```python
from build123d import *

# Parameters (mm, degrees)
SKETCH1_W           = 25.4
SKETCH1_H           = 38.1
BOSS_EXTRUDE1_DEPTH = 152.4
SHELL1_T            = -3.175
SKETCH2_R           = 9.525
CUT_EXTRUDE1_DEPTH  = 156.672163536
SKETCH3_R           = 2.38125
CUT_EXTRUDE2_DEPTH  = 158.602855304
SKETCH4_R           = 2.38125
CUT_EXTRUDE3_DEPTH  = 156.672163536
SKETCH5_R           = 2.38125
CUT_EXTRUDE4_DEPTH  = 158.602855304


with BuildPart() as part:
    # Sketch1 → Boss-Extrude1 (new body)
    with BuildSketch(Plane.XY):
        Rectangle(SKETCH1_W, SKETCH1_H)
    extrude(amount=BOSS_EXTRUDE1_DEPTH)

    # Shell1
    shell1_openings = [part.faces().sort_by_distance(p)[0] for p in [
        (0, 0, 152.4),
        (0, 0, 0),
    ]]
    offset(amount=SHELL1_T, openings=shell1_openings, kind=Kind.INTERSECTION)

    # Sketch2 → Cut-Extrude1 (cut, through all)
    with BuildSketch(Plane(origin=(12.7, 0, 0), x_dir=(0, 0, -1), z_dir=(1, 0, 0))):
        with Locations((-53.975, -12.7)):
            Circle(SKETCH2_R)
    extrude(amount=-CUT_EXTRUDE1_DEPTH, mode=Mode.SUBTRACT)

    # Sketch3 → Cut-Extrude2 (cut, through all)
    with BuildSketch(Plane(origin=(0, 19.05, 0), x_dir=(1, 0, 0), z_dir=(0, 1, 0))):
        with Locations(Location((0, -139.7, 0), (0, 0, 270))):
            Circle(SKETCH3_R)
        with Locations(Location((0, -114.3, 0), (0, 0, 270))):
            Circle(SKETCH3_R)
    extrude(amount=-CUT_EXTRUDE2_DEPTH, mode=Mode.SUBTRACT)

    # Sketch4 → Cut-Extrude3 (cut, through all)
    with BuildSketch(Plane(origin=(12.7, 0, 0), x_dir=(0, 0, -1), z_dir=(1, 0, 0))):
        with Locations(Location((-79.375, -9.525, 0), (0, 0, 90))):
            Circle(SKETCH4_R)
        with Locations(Location((-104.775, -9.525, 0), (0, 0, 90))):
            Circle(SKETCH4_R)
    extrude(amount=-CUT_EXTRUDE3_DEPTH, mode=Mode.SUBTRACT)

    # Sketch5 → Cut-Extrude4 (cut, through all)
    with BuildSketch(Plane(origin=(0, 19.05, 0), x_dir=(1, 0, 0), z_dir=(0, 1, 0))):
        with Locations(Location((0, -12.7, 0), (0, 0, 270))):
            Circle(SKETCH5_R)
        with Locations(Location((0, -38.1, 0), (0, 0, 270))):
            Circle(SKETCH5_R)
    extrude(amount=-CUT_EXTRUDE4_DEPTH, mode=Mode.SUBTRACT)


solid = part.part
```
Read the model definition and answer for the solid it produces. Units are mm, in the model's axes. A direction names the side the tool comes from. Give positions to 0.01 mm unless a question says otherwise; leave off trailing zeros. Loops run counter-clockwise (first coordinate to the right, second up) from the corner with the lowest first, then second, coordinate; pieces in that order, holes last.
Item 1: The part is cut by section C-C (y = 11.5). Write down the section's boundary in (x, z) (3 decimals).
Item 2: The part is cut by section D-D (y = -9.5). Give the number of separate pieces and of enclosed holes in the cut face, and give its area (3 significant figures).
Item 3: Find the intervals of material crossed by line 1 along X through (y, z) = (14, 61) (3 decimals); line 2 along Y through (x, z) = (-9, 67) (3 decimals); line 3 along X through (y, z) = (17, 38), in increasing order.
Item 4: The part is cut by section B-B (x = 8.25). Write down the section's boundary in (y, z) (3 decimals), and give its area (3 significant figures).
Item 5: The part is cut by section A-A (z = 12.7). Write down the section's boundary in (x, y) (3 decimals), and give its area (3 significant figures).
Item 6: Each of these flat-tipped pins is pushed along its axis until it touches: pin 1 Ø4 at (y, z) = (-9.525, 104.775) entering from -X; pin 2 Ø9.5 at (x, z) = (-1.5, 52) entering from -Y (3 decimals). Where does it stop, or does it pass through?
Item 7: For faces 4 (the cylindrical face through (-0.91, -17.44, 40.3)), 5 (the flat face through (9.525, 0, 75)), determine the directions among +Z, -Z, +X, -X, +Y, -Y from which every point of the face is accessible in a straight line to the end or side of a thin tool.
Item 8: The mould has two halves that part along Z. Classify faces 1 (the flat face through (0, 15.875, 75)), 2 (the cylindrical face through (-0.91, 17.48, 116.5)), 3 (the flat face through (11, 0, 152.4)): released by +Z, released by -Z, zero draft, split by the parting line, or undercut.
Taken from the geometry:
1. outline: (-12.7, 0) - (-9.525, 0) - (-9.525, 152.4) - (-12.7, 152.4) - close; (9.525, 0) - (12.7, 0) - (12.7, 152.4) - (9.525, 152.4) - close
2. separate pieces: 8
2. enclosed holes: 0
2. area: 793 mm2
3. line 1: x = -12.7 to -9.525, 9.525 to 12.7
3. line 2: y = -19.05 to -15.875, 15.875 to 19.05
3. line 3: x = -12.7 to -2.38, 2.38 to 12.7
4. outline: (-19.05, 0) - (-15.875, 0) - (-15.875, 44.995) arc R9.525 cw to (-19.05, 46.875) - close; (-19.05, 61.075) arc R9.525 cw to (-15.875, 62.955) - (-15.875, 152.4) - (-19.05, 152.4) - close; (15.875, 0) - (19.05, 0) - (19.05, 152.4) - (15.875, 152.4) - close
4. area: 916 mm2
5. outline: (-12.7, -19.05) - (-2.381, -19.05) - (-2.381, -15.875) - (-9.525, -15.875) - (-9.525, 15.875) - (-2.381, 15.875) - (-2.381, 19.05) - (-12.7, 19.05) - close; (2.381, -19.05) - (12.7, -19.05) - (12.7, 19.05) - (2.381, 19.05) - (2.381, 15.875) - (9.525, 15.875) - (9.525, -15.875) - (2.381, -15.875) - close
5. area: 333 mm2
6. pin 1: passes through
6. pin 2: stops at y = 15.875
7. face 4: +Y, -Y
7. face 5: +Z, -Z
8. face 1: zero draft
8. face 2: undercut
8. face 3: released by +Z
